from build123d import *

# Parameters (mm, degrees)
SKETCH_1_R          = 35
SKETCH_1_R_2        = 19
SKETCH_1_R_3        = 2
EXTRUDE_1_DEPTH     = 5
SKETCH_2_R          = 3.75
CUT_EXTRUDE_1_DEPTH = 2.5


with BuildPart() as part:
    # 草图1 → 凸台-拉伸1 (new body)
    with BuildSketch(Plane(origin=(0, 0, 0), x_dir=(1, 0, 0), z_dir=(0, 1, 0))):
        with Locations(Location((0, 0, 0), (0, 0, 270))):
            Circle(SKETCH_1_R)
        with Locations(Location((0, 0, 0), (0, 0, 270))):
            Circle(SKETCH_1_R_2, mode=Mode.SUBTRACT)
        with Locations(Location((0, 30, 0), (0, 0, 270))):
            Circle(SKETCH_1_R_3, mode=Mode.SUBTRACT)
        with Locations(Location((25.980762114, 15, 0), (0, 0, 270))):
            Circle(SKETCH_1_R_3, mode=Mode.SUBTRACT)
        with Locations(Location((25.980762114, -15, 0), (0, 0, 270))):
            Circle(SKETCH_1_R_3, mode=Mode.SUBTRACT)
        with Locations(Location((0, -30, 0), (0, 0, 270))):
            Circle(SKETCH_1_R_3, mode=Mode.SUBTRACT)
        with Locations(Location((-25.980762114, -15, 0), (0, 0, 270))):
            Circle(SKETCH_1_R_3, mode=Mode.SUBTRACT)
        with Locations(Location((-25.980762114, 15, 0), (0, 0, 270))):
            Circle(SKETCH_1_R_3, mode=Mode.SUBTRACT)
    extrude(amount=EXTRUDE_1_DEPTH)

    # 草图2 → 切除-拉伸1 (cut)
    with BuildSketch(Plane.XZ):
        with Locations(Location((0, 30, 0), (0, 0, 270))):
            Circle(SKETCH_2_R)
        with Locations(Location((25.980762114, 15, 0), (0, 0, 270))):
            Circle(SKETCH_2_R)
        with Locations(Location((25.980762114, -15, 0), (0, 0, 270))):
            Circle(SKETCH_2_R)
        with Locations(Location((0, -30, 0), (0, 0, 270))):
            Circle(SKETCH_2_R)
        with Locations(Location((-25.980762114, -15, 0), (0, 0, 270))):
            Circle(SKETCH_2_R)
        with Locations(Location((-25.980762114, 15, 0), (0, 0, 270))):
            Circle(SKETCH_2_R)
    extrude(amount=-CUT_EXTRUDE_1_DEPTH, mode=Mode.SUBTRACT)


solid = part.part
Build history of the part. All positions in model axes, mm. A direction names the side the tool comes from. Round coordinates to 2 decimals unless told otherwise and drop trailing zeros. Write each loop counter-clockwise with the first axis right and the second up, starting at its lowest first coordinate (ties: lowest second). Pieces come first, ordered by that corner, then holes. Notation, with made-up numbers: M 40,32 L 71,32 A10 ccw 71,45 Z; hole C 32,57.5 d2. An arc over 180 degrees is marked long. Answer in a Markdown table with one row per item.
1. Saw through at B-B (x = 12). List the corners of the cut face in (y, z).
Geometry check:
| item | result |
|---|---|
| outline | M 0,-32.88 L 5,-32.88 L 5,-14.73 L 0,-14.73 Z; M 0,14.73 L 5,14.73 L 5,32.88 L 0,32.88 Z |
2. Saw through at C-C (x = 0). List the corners of the cut face in (y, z), and give its area (4 significant figures).
Geometry check:
| item | result |
|---|---|
| outline | M 0,-35 L 5,-35 L 5,-32 L 2.5,-32 L 2.5,-33.75 L 0,-33.75 Z; M 0,-26.25 L 2.5,-26.25 L 2.5,-28 L 5,-28 L 5,-19 L 0,-19 Z; M 0,19 L 5,19 L 5,28 L 2.5,28 L 2.5,26.25 L 0,26.25 Z; M 0,33.75 L 2.5,33.75 L 2.5,32 L 5,32 L 5,35 L 0,35 Z |
| area | 102.5 mm2 |
3. Which spindle directions (+Z, -Z, +X, -X, +Y, -Y) get a long thin tool onto all of the face, cutting with end or side? Do faces 4 (the face through (-27.755, 3.732, -14.077)), 5 (the face through (0.165, 1.232, -26.254)). Say none if no direction does.
Geometry check:
| item | result |
|---|---|
| face 4 | +Y, -Y |
| face 5 | -Y |
4. Flat gauge pins, fed straight in: P1, Ø2, axis at x = 16.5, y = 2.5, coming from the -Z side; P2, Ø1, axis at x = -18, y = 1.5, coming from the +Z side; P3, Ø3, axis at y = 3, z = 13.5, coming from the +X side. Where does each tip first touch, or does it go through?
Geometry check:
| item | result |
|---|---|
| P1 | z = -31.38 |
| P2 | z = 30.31 |
| P3 | x = 32.88 |
5. Saw through at D-D (y = 0.85). List the corners of the cut face in (x, z).
Geometry check:
| item | result |
|---|---|
| outline | C 0,0 d70; hole C -25.98,-15 d7.5; hole C -25.98,15 d7.5; hole C 0,0 d38; hole C 0,-30 d7.5; hole C 0,30 d7.5; hole C 25.98,-15 d7.5; hole C 25.98,15 d7.5 |
6. Saw through at A-A (z = 0). List the corners of the cut face in (x, y), and give its area (3 significant figures).
Geometry check:
| item | result |
|---|---|
| outline | M -35,0 L -19,0 L -19,5 L -35,5 Z; M 19,0 L 35,0 L 35,5 L 19,5 Z |
| area | 160 mm2 |
7. Mould opens along X. For faces 1 (the face through (-21, 2, -28)), 2 (the face through (-15, 5, 15)), 3 (the face through (-0.766, 3.732, 31.847)) say: +X half, -X half, draft (parallel to the pull), parting line (faces both ways), or undercut.
Geometry check:
| item | result |
|---|---|
| face 1 | parting line |
| face 2 | draft |
| face 3 | undercut |
8. Probe L1, parallel to Z at x = -26, y = 0.6; L2, parallel to Z at x = 1.5, y = 1.15; L3, parallel to Z at x = -6, y = 1.75. List the from-to ranges inside material, lowest first. Write a range as [from, to].
Geometry check:
| item | result |
|---|---|
| L1 | [-23.43, -18.75], [-11.25, 11.25], [18.75, 23.43] |
| L2 | [-34.97, -33.44], [-26.56, -18.94], [18.94, 26.56], [33.44, 34.97] |
| L3 | [-34.48, -18.03], [18.03, 34.48] |
